Verification items for the finished model (mm, model axes). Face numbers are marked on the shaded views. A direction names the side the tool comes from. Give positions to 0.01 mm unless a question says otherwise; leave off trailing zeros. Write each loop counter-clockwise with the first axis right and the second up, starting at its lowest first coordinate (ties: lowest second). Pieces come first, ordered by that corner, then holes. Notation, with made-up numbers: (0.5, 34) -> (23.5, 34) arc R10 ccw to (23.5, 49) -> close; hole circle Ø9 at (25.25, -19). An arc over 180 degrees is marked (long way). Answer as CSV lines item,"result".
```python
from build123d import *

# Parameters (mm, degrees)
MIDBODYS_R                   = 3
MIDBODY_DEPTH                = 0.8
MIDORINGBODYS_R              = 2.5
MIDORINGBODY_DEPTH           = 0.6
EXTENDEDMIDBODYS_R           = 2.5
EXTENDEDMIDBODY_DEPTH        = 7.6
F_2NDORINGBODYS_R            = 2.5
F_2NDORINGBODY_DEPTH         = 0.6
F_2NDEXTENDEDBODYS_R         = 3
F_2NDEXTENDEDBODY_DEPTH      = 4.5
F_3RDORINGBODYS_R            = 2.5
F_3RDORINGBODY_DEPTH         = 0.8
ENDBODY_START                = 4.6
ENDBODYS_R                   = 3.6
ENDBODY_DEPTH                = 4.6
F_4_0_4_DIAMETER_HOLE1_D     = 4
F_4_0_4_DIAMETER_HOLE1_DEPTH = 9.4
F_4_0_4_DIAMETER_HOLE1_TIP   = 1.201721238


with BuildPart() as part:
    # MidBodyS → MidBody (new body)
    with BuildSketch(Plane(origin=(0, 0, 0), x_dir=(1, 0, 0), z_dir=(0, 1, 0))):
        with Locations(Location((0, 0, 0), (0, 0, 270))):
            Circle(MIDBODYS_R)
    midbody = extrude(amount=MIDBODY_DEPTH)

    # MidORingBaseS → MidORingBase (revolve)
    with BuildSketch(Plane.XY, mode=Mode.PRIVATE) as midoringbase_sk:
        Polygon((3, 0.8), (3.6, 1.3), (3.6, 1.6), (0, 1.6), (0, 0.8), align=None)
    midoringbase = revolve(midoringbase_sk.sketch.rotate(Axis((0, 1.6, 0), (0, -1, 0)), 180), axis=Axis((0, 1.6, 0), (0, -1, 0)))

    # MidORingBodyS → MidORingBody (add)
    with BuildSketch(Plane(origin=(0, 1.6, 0), x_dir=(1, 0, 0), z_dir=(0, 1, 0))):
        with Locations(Location((0, 0, 0), (0, 0, 180))):
            Circle(MIDORINGBODYS_R)
    midoringbody = extrude(amount=MIDORINGBODY_DEPTH)

    # MidORingTopBaseS → MidORingTopBase (revolve)
    with BuildSketch(Plane.XY, mode=Mode.PRIVATE) as midoringtopbase_sk:
        Polygon((0, 2.2), (3.6, 2.2), (3.6, 2.5), (2.5, 3), (0, 3), align=None)
    midoringtopbase = revolve(midoringtopbase_sk.sketch.rotate(Axis((0, 2.2, 0), (0, 1, 0)), 90), axis=Axis((0, 2.2, 0), (0, 1, 0)))

    # ExtendedMidBodyS → ExtendedMidBody (add)
    with BuildSketch(Plane(origin=(0, 3, 0), x_dir=(1, 0, 0), z_dir=(0, 1, 0))):
        with Locations(Location((0, 0, 0), (0, 0, 180))):
            Circle(EXTENDEDMIDBODYS_R)
    extendedmidbody = extrude(amount=EXTENDEDMIDBODY_DEPTH)

    # 2ndORingBaseS → 2ndORingBase (revolve)
    with BuildSketch(Plane.XY):
        Polygon((0, 11.4), (3.6, 11.4), (3.6, 11.1), (2.5, 10.6), (0, 10.6), align=None)
    f_2ndoringbase = revolve(axis=Axis((0, 10.6, 0), (0, 1, 0)))

    # 2ndORingBodyS → 2ndORingBody (add)
    with BuildSketch(Plane(origin=(0, 11.4, 0), x_dir=(1, 0, 0), z_dir=(0, 1, 0))):
        with Locations(Location((0, 0, 0), (0, 0, 180))):
            Circle(F_2NDORINGBODYS_R)
    f_2ndoringbody = extrude(amount=F_2NDORINGBODY_DEPTH)

    # 2ndORingBaseTopS → 2ndORingBaseTop (revolve)
    with BuildSketch(Plane.XY, mode=Mode.PRIVATE) as f_2ndoringbasetop_sk:
        Polygon((0, 12), (3.6, 12), (3.6, 12.3), (3, 12.8), (0, 12.8), align=None)
    f_2ndoringbasetop = revolve(f_2ndoringbasetop_sk.sketch.rotate(Axis((0, 12.8, 0), (0, -1, 0)), 180), axis=Axis((0, 12.8, 0), (0, -1, 0)))

    # 2ndExtendedBodyS → 2ndExtendedBody (add)
    with BuildSketch(Plane(origin=(0, 12.8, 0), x_dir=(1, 0, 0), z_dir=(0, 1, 0))):
        with Locations(Location((0, 0, 0), (0, 0, 270))):
            Circle(F_2NDEXTENDEDBODYS_R)
    f_2ndextendedbody = extrude(amount=F_2NDEXTENDEDBODY_DEPTH)

    # 3rdORingBaseS → 3rdORingBase (revolve)
    with BuildSketch(Plane.XY, mode=Mode.PRIVATE) as f_3rdoringbase_sk:
        Polygon((0, 17.3), (3, 17.3), (3.6, 17.8), (3.6, 18.1), (0, 18.1), align=None)
    f_3rdoringbase = revolve(f_3rdoringbase_sk.sketch.rotate(Axis((0, 18.1, 0), (0, -1, 0)), 180), axis=Axis((0, 18.1, 0), (0, -1, 0)))

    # 3rdORingBodyS → 3rdORingBody (add)
    with BuildSketch(Plane(origin=(0, 18.1, 0), x_dir=(1, 0, 0), z_dir=(0, 1, 0))):
        with Locations(Location((0, 0, 0), (0, 0, 180))):
            Circle(F_3RDORINGBODYS_R)
    f_3rdoringbody = extrude(amount=F_3RDORINGBODY_DEPTH)

    # EndBodyS → EndBody (add)
    with BuildSketch(Plane(origin=(0, 18.9, 0), x_dir=(1, 0, 0), z_dir=(0, 1, 0)).offset(ENDBODY_START)):
        with Locations(Location((0, 0, 0), (0, 0, 180))):
            Circle(ENDBODYS_R)
    endbody = extrude(amount=-ENDBODY_DEPTH)

    # HalfBodyVM: MidBody, MidORingBase, MidORingBody, MidORingTopBase, ExtendedMidBody, 2ndORingBase, 2ndORingBody, 2ndORingBaseTop, 2ndExtendedBody, 3rdORingBase, 3rdORingBody, EndBody across plane
    add(midbody.mirror(Plane.ZX))
    add(midoringbase.mirror(Plane.ZX))
    add(midoringbody.mirror(Plane.ZX))
    add(midoringtopbase.mirror(Plane.ZX))
    add(extendedmidbody.mirror(Plane.ZX))
    add(f_2ndoringbase.mirror(Plane.ZX))
    add(f_2ndoringbody.mirror(Plane.ZX))
    add(f_2ndoringbasetop.mirror(Plane.ZX))
    add(f_2ndextendedbody.mirror(Plane.ZX))
    add(f_3rdoringbase.mirror(Plane.ZX))
    add(f_3rdoringbody.mirror(Plane.ZX))
    add(endbody.mirror(Plane.ZX))

    # Ø4.0 (4) Diameter Hole1
    with Locations(Plane(origin=(0, -23.5, 0), x_dir=(-1, 0, 0), z_dir=(0, -1, 0))):
        with Locations((0, 0)):
            Hole(F_4_0_4_DIAMETER_HOLE1_D / 2, depth=F_4_0_4_DIAMETER_HOLE1_DEPTH)
            with Locations((0, 0, -(F_4_0_4_DIAMETER_HOLE1_DEPTH + F_4_0_4_DIAMETER_HOLE1_TIP / 2))):  # 118° drill point
                Cone(0, F_4_0_4_DIAMETER_HOLE1_D / 2, F_4_0_4_DIAMETER_HOLE1_TIP, mode=Mode.SUBTRACT)


solid = part.part
```
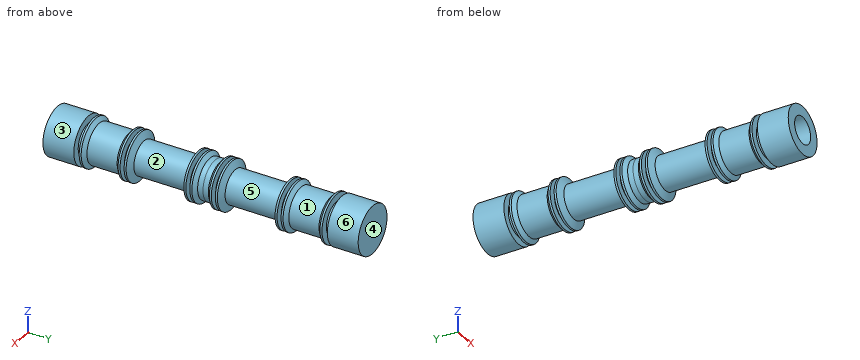
1) Depth check by flat-ended pin: pin 1 (2.5 mm diameter, centred on x = 0, z = 0, fed in from -Y). Enter the tip coordinate at first touch or a pass-through.
Reported:
pin 1,"y = -13.65"
2) Tool access check on the marked faces 5 and 6. Record the directions out of +Z, -Z, +X, -X, +Y, -Y that give a thin tool (end or side, any length) a straight path to the whole face; none if there is none.
Reported:
face 5,"none"
face 6,"+Y, -Y"
3) Draft check along Y on the marked faces 1, 2, 3 and 4. Enter one of: +Y half, -Y half, draft (parallel to the pull), parting line (faces both ways), or undercut.
Reported:
face 1,"undercut"
face 2,"undercut"
face 3,"draft"
face 4,"+Y half"
4) Scan lines: line 1 along Z through (x, y) = (0, -21.25); line 2 along Z through (x, y) = (0, -17.75); line 3 along X through (y, z) = (9, 1.5). Record each from-to range of solid material in increasing order.
Reported:
line 1,"-3.6 to -2, 2 to 3.6"
line 2,"-3.54 to -2, 2 to 3.54"
line 3,"-2 to 2"
5) Section check A-A (y = 19.5). Record the boundary of the cut face in (x, z), and give its area (3 significant figures).
Reported:
outline,"circle Ø7.2 at (0, 0)"
area,"40.7 mm²"
